Study the drawing (mm; zero at the part's minimum x, y, z) and answer. Round coordinates to 2 decimals unless told otherwise and drop trailing zeros. Loops run counter-clockwise (first coordinate to the right, second up) from the corner with the lowest first, then second, coordinate; pieces in that order, holes last. Notation, with made-up numbers: (-26, 36.5) -> (11, 36.5) arc R37 ccw to (11, 73.5) -> close; hole circle Ø9 at (70, 4.5). An arc over 180 degrees is marked (long way). Use one line per item in the form item = value.
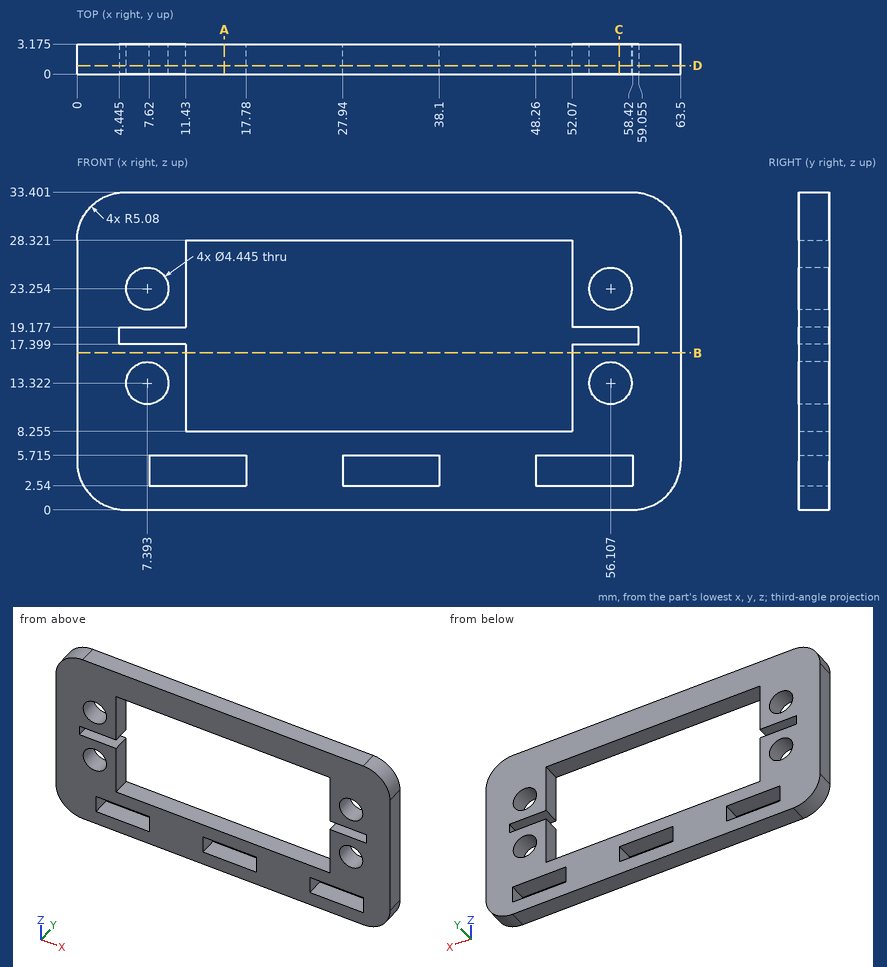
(1) Find section D-D, the plane y = 0.9. State how many separate pieces and enclosed holes the cut face has, then the cut area to 3 significant figures.
Completed:
separate_pieces = 1
enclosed_holes = 8
area = 1,100 mm2
(2) Consider L1, parallel to Z at x = 32.5, y = 1.45 (1 decimal); L2, parallel to X at y = 1.4, z = 5; L3, parallel to X at y = 0.4, z = 23.5. Determine where each line is inside the solid, lowest interval first.
Completed:
L1 = 0 to 2.5, 5.7 to 8.3, 28.3 to 33.4
L2 = 0 to 7.62, 17.78 to 27.94, 38.1 to 48.26, 58.42 to 63.5
L3 = 0 to 5.18, 9.6 to 11.43, 52.07 to 53.9, 58.32 to 63.5
(3) Find section C-C, the plane x = 57. Write down the section's boundary in (y, z) (1 decimal).
Completed:
outline = (0, 0) -> (3.2, 0) -> (3.2, 2.5) -> (0, 2.5) -> close; (0, 5.7) -> (3.2, 5.7) -> (3.2, 11.3) -> (0, 11.3) -> close; (0, 15.4) -> (3.2, 15.4) -> (3.2, 17.4) -> (0, 17.4) -> close; (0, 19.2) -> (3.2, 19.2) -> (3.2, 21.2) -> (0, 21.2) -> close; (0, 25.3) -> (3.2, 25.3) -> (3.2, 33.4) -> (0, 33.4) -> close
(4) Find section A-A, the plane x = 15.5. Write down the section's boundary in (y, z) (1 decimal).
Completed:
outline = (0, 0) -> (3.2, 0) -> (3.2, 2.5) -> (0, 2.5) -> close; (0, 5.7) -> (3.2, 5.7) -> (3.2, 8.3) -> (0, 8.3) -> close; (0, 28.3) -> (3.2, 28.3) -> (3.2, 33.4) -> (0, 33.4) -> close
(5) Find section B-B, the plane z = 16.5. Write down the section's boundary in (x, y) (1 decimal).
Completed:
outline = (0, 0) -> (11.4, 0) -> (11.4, 3.2) -> (0, 3.2) -> close; (52.1, 0) -> (63.5, 0) -> (63.5, 3.2) -> (52.1, 3.2) -> close
